```python
from build123d import *

# Parameters (mm, degrees)
F1_DEPTH      = 101.6
F3_DEPTH      = 287
F3_DEPTH_BACK = 50.801
F5_DEPTH      = 3.81


# Not quite as in the source:
# - an extrude ends at something that could not be found from the text; its depth is read off the source's solid


with BuildPart() as f1:
    # F0 (on Top) → F1 (new body, symmetric)
    with BuildSketch(Plane.XY):
        Polygon((44.45, 101.6), (44.45, 6.35), (0, 6.35), (0, 0), (50.8, 0), (50.8, 101.6), align=None)
    extrude(amount=F1_DEPTH, both=True)

    # F2 (on Right) → F3 (cut, two sides)
    with BuildSketch(Plane.YZ) as f3_sk:
        with BuildLine():
            ThreePointArc((47.625, -73.025), (48.5549359697, -75.2700640303), (50.8, -76.2))
            ThreePointArc((50.8, -76.2), (53.0450640303, -75.2700640303), (53.975, -73.025))
            Line((53.975, -73.025), (53.975, 73.0249999165))
            ThreePointArc((53.975, 73.0249999165), (53.0450640598, 75.2700640008), (50.8, 76.2))
            ThreePointArc((50.8, 76.2), (48.5549359697, 75.2700640303), (47.625, 73.025))
            Line((47.625, 73.025), (47.625, -73.025))
        make_face()
    extrude(amount=-F3_DEPTH, mode=Mode.SUBTRACT)
    extrude(f3_sk.sketch, amount=F3_DEPTH_BACK, mode=Mode.SUBTRACT)

    # F4 (on face) → F5 (cut)
    with BuildSketch(Plane.YZ.offset(50.8)):
        with BuildLine():
            Line((54.7984857559, -73.5657372472), (54.7984857559, 73.7838448219))
            ThreePointArc((54.7984857559, 73.7838448219), (50.7384735742, 77.6595205582), (46.8004034081, 73.66))
            Line((46.8004034081, 73.66), (46.8004034081, -73.740335956))
            ThreePointArc((46.8004034081, -73.740335956), (50.8868960802, -77.6590472365), (54.7984857559, -73.5657372472))
        make_face()
    extrude(amount=-F5_DEPTH, mode=Mode.SUBTRACT)

    # F6: F1 across plane


with BuildPart() as f1_1:
    add(f1.part)
    add(f1.part.mirror(Plane.YZ))


solid = f1_1.part
```
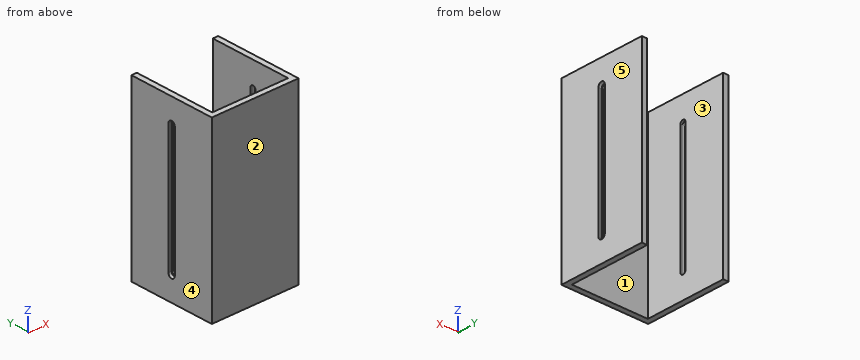
Input: part model. Units: mm. Frame: model coordinates. Face numbers are marked on the shaded views. A direction names the side the tool comes from. Round coordinates to 2 decimals unless told otherwise and drop trailing zeros. Order: outer loops, then holes, each group sorted by start corner. A loop starts at its lowest first (then second) coordinate and runs counter-clockwise, first axis right, second up. Notation, with made-up numbers: (-5.75, 15.5) - (41.25, 15.5) arc R16 cw to (41.25, 36.5) - close; hole circle Ø7 at (-8, 88.25). An arc over 180 degrees is marked (long way). One line per question, with ' | ' between items. Start each with the question number.
1) Ray query, probe 1 along X at (y, z) = (35, -83); probe 2 along Y at (x, z) = (-14.5, -24). Return the intervals inside material, ascending.
2) Pull-direction query (X, two-part tool) for the marked faces 3, 4 and 5; classes: +X half, -X half, draft (parallel to the pull), parting line (faces both ways), or undercut.
3) Cut plane C-C, the plane x = 20. Return the cut outline in (y, z).
4) Cut plane B-B, the plane z = 3. Return the cut outline in (x, y) (3 decimals), then the cut area to 3 significant figures.
5) Cut plane A-A, the plane y = 88. Return the cut outline in (x, z), then the cut area to 3 significant figures.
6) Contact query for flat-ended pins moving along their axis: P1, Ø12, axis at x = 34.5, z = -61.5, coming from the -Y side; P2, Ø6, axis at x = 18, z = 79.5, coming from the +Y side; P3, Ø2.5, axis at y = 51, z = -29, coming from the -X side. Output: stop coordinate, or through.
7) Set-up query: the marked faces 1 and 2. Return all of +Z, -Z, +X, -X, +Y, -Y with unobstructed straight access to the full face (end or side cutting, diameter ignored); none if empty.
Worked out:
1) probe 1: x = -50.8 to -44.45, 44.45 to 50.8 | probe 2: y = 0 to 6.35
2) face 3: undercut | face 4: -X half | face 5: +X half
3) outline: (0, -101.6) - (6.35, -101.6) - (6.35, 101.6) - (0, 101.6) - close
4) outline: (-50.8, 0) - (50.8, 0) - (50.8, 46.8) - (46.99, 46.8) - (46.99, 47.625) - (44.45, 47.625) - (44.45, 6.35) - (-44.45, 6.35) - (-44.45, 47.625) - (-46.99, 47.625) - (-46.99, 46.8) - (-50.8, 46.8) - close; (-50.8, 54.798) - (-46.99, 54.798) - (-46.99, 53.975) - (-44.45, 53.975) - (-44.45, 101.6) - (-50.8, 101.6) - close; (44.45, 53.975) - (46.99, 53.975) - (46.99, 54.798) - (50.8, 54.798) - (50.8, 101.6) - (44.45, 101.6) - close | area: 1,760 mm^2
5) outline: (-50.8, -101.6) - (-44.45, -101.6) - (-44.45, 101.6) - (-50.8, 101.6) - close; (44.45, -101.6) - (50.8, -101.6) - (50.8, 101.6) - (44.45, 101.6) - close | area: 2,580 mm^2
6) P1: stops at y = 0 | P2: stops at y = 6.35 | P3: passes through
7) face 1: +Z, -Z, +Y | face 2: +Z, -Z, +X, -X, -Y
